```python
from build123d import *

# Parameters (mm, degrees)
SZKIC1_W = 9
SZKIC1_H = 21
SZKIC3_W = 1.2
SZKIC3_H = 2.1
SZKIC4_W = 6
SZKIC4_H = 23.5
SZKIC5_W = 40
SZKIC5_H = 21
SZKIC6_W = 1.2
SZKIC6_H = 2.1
SZKIC8_W = 165
SZKIC8_H = 16
SZKIC9_W = 1.2
SZKIC9_H = 1.6


with BuildPart() as part:
    # Szkic1 → Obr_t1 (revolve)
    with BuildSketch(Plane(origin=(0, 0, 0), x_dir=(0, 0, -1), z_dir=(1, 0, 0)), mode=Mode.PRIVATE) as obr_t1_sk:
        with Locations((-4.5, 10.5)):
            Rectangle(SZKIC1_W, SZKIC1_H)
    revolve(obr_t1_sk.sketch.rotate(Axis((0, 0, 0), (0, 0, 1)), 270), axis=Axis((0, 0, 0), (0, 0, 1)))

    # Szkic2 → Wyci_cie-obr_t1 (revolve, cut)
    with BuildSketch(Plane(origin=(0, 0, 0), x_dir=(0, 0, -1), z_dir=(1, 0, 0)), mode=Mode.PRIVATE) as wyci_cie_obr_t1_sk:
        Polygon((-0.707106781, 21), (0, 20.292893219), (0, 21), align=None)
    revolve(wyci_cie_obr_t1_sk.sketch.rotate(Axis((0, 0, 0), (0, 0, 1)), 270), axis=Axis((0, 0, 0), (0, 0, 1)), mode=Mode.SUBTRACT)

    # Szkic3 → Wyci_cie-obr_t2 (revolve, cut)
    with BuildSketch(Plane(origin=(0, 0, 0), x_dir=(0, 0, -1), z_dir=(1, 0, 0)), mode=Mode.PRIVATE) as wyci_cie_obr_t2_sk:
        with Locations((-8.4, 19.95)):
            Rectangle(SZKIC3_W, SZKIC3_H)
    revolve(wyci_cie_obr_t2_sk.sketch.rotate(Axis((0, 0, 0), (0, 0, 1)), 270), axis=Axis((0, 0, 0), (0, 0, 1)), mode=Mode.SUBTRACT)

    # Szkic4 → Obr_t2 (revolve)
    with BuildSketch(Plane(origin=(0, 0, 0), x_dir=(0, 0, -1), z_dir=(1, 0, 0)), mode=Mode.PRIVATE) as obr_t2_sk:
        with Locations((-12, 11.75)):
            Rectangle(SZKIC4_W, SZKIC4_H)
    revolve(obr_t2_sk.sketch.rotate(Axis((0, 0, 9), (0, 0, 1)), 270), axis=Axis((0, 0, 9), (0, 0, 1)))

    # Szkic5 → Obr_t3 (revolve)
    with BuildSketch(Plane(origin=(0, 0, 0), x_dir=(0, 0, -1), z_dir=(1, 0, 0)), mode=Mode.PRIVATE) as obr_t3_sk:
        with Locations((-35, 10.5)):
            Rectangle(SZKIC5_W, SZKIC5_H)
    revolve(obr_t3_sk.sketch.rotate(Axis((0, 0, 15), (0, 0, 1)), 270), axis=Axis((0, 0, 15), (0, 0, 1)))

    # Szkic6 → Wyci_cie-obr_t3 (revolve, cut)
    with BuildSketch(Plane(origin=(0, 0, 0), x_dir=(0, 0, -1), z_dir=(1, 0, 0)), mode=Mode.PRIVATE) as wyci_cie_obr_t3_sk:
        with Locations((-15.6, 19.95)):
            Rectangle(SZKIC6_W, SZKIC6_H)
    revolve(wyci_cie_obr_t3_sk.sketch.rotate(Axis((0, 0, 15), (0, 0, 1)), 270), axis=Axis((0, 0, 15), (0, 0, 1)), mode=Mode.SUBTRACT)

    # Szkic7 → Wyci_cie-obr_t4 (revolve, cut)
    with BuildSketch(Plane(origin=(0, 0, 0), x_dir=(0, 0, -1), z_dir=(1, 0, 0)), mode=Mode.PRIVATE) as wyci_cie_obr_t4_sk:
        Polygon((-55, 20.292893219), (-54.292893219, 21), (-55, 21), align=None)
    revolve(wyci_cie_obr_t4_sk.sketch.rotate(Axis((0, 0, 9), (0, 0, 1)), 270), axis=Axis((0, 0, 9), (0, 0, 1)), mode=Mode.SUBTRACT)

    # Szkic8 → Obr_t4 (revolve)
    with BuildSketch(Plane(origin=(0, 0, 0), x_dir=(0, 0, -1), z_dir=(1, 0, 0)), mode=Mode.PRIVATE) as obr_t4_sk:
        with Locations((-137.5, 8)):
            Rectangle(SZKIC8_W, SZKIC8_H)
    revolve(obr_t4_sk.sketch.rotate(Axis((0, 0, 55), (0, 0, 1)), 270), axis=Axis((0, 0, 55), (0, 0, 1)))

    # Szkic9 → Wyci_cie-obr_t5 (revolve, cut)
    with BuildSketch(Plane(origin=(0, 0, 0), x_dir=(0, 0, -1), z_dir=(1, 0, 0)), mode=Mode.PRIVATE) as wyci_cie_obr_t5_sk:
        with Locations((-55.6, 15.2)):
            Rectangle(SZKIC9_W, SZKIC9_H)
    revolve(wyci_cie_obr_t5_sk.sketch.rotate(Axis((0, 0, 55), (0, 0, 1)), 270), axis=Axis((0, 0, 55), (0, 0, 1)), mode=Mode.SUBTRACT)

    # Szkic10 → Wyci_cie-obr_t6 (revolve, cut)
    with BuildSketch(Plane(origin=(0, 0, 0), x_dir=(0, 0, -1), z_dir=(1, 0, 0)), mode=Mode.PRIVATE) as wyci_cie_obr_t6_sk:
        Polygon((-220, 14.124355653), (-213, 16), (-220, 16), align=None)
    revolve(wyci_cie_obr_t6_sk.sketch.rotate(Axis((0, 0, 55), (0, 0, 1)), 270), axis=Axis((0, 0, 55), (0, 0, 1)), mode=Mode.SUBTRACT)

    # Szkic11 → Wyci_cie-obr_t7 (revolve, cut)
    with BuildSketch(Plane(origin=(0, 0, 0), x_dir=(0, 0, -1), z_dir=(1, 0, 0)), mode=Mode.PRIVATE) as wyci_cie_obr_t7_sk:
        with BuildLine():
            Line((-218.332342851, 14.571203039), (-220, 14.124355653))
            Line((-220, 14.124355653), (-220, 12.39786993))
            ThreePointArc((-220, 12.39786993), (-219.535045016, 13.767583145), (-218.332342851, 14.571203039))
        make_face()
    revolve(wyci_cie_obr_t7_sk.sketch.rotate(Axis((0, 0, 55), (0, 0, 1)), 270), axis=Axis((0, 0, 55), (0, 0, 1)), mode=Mode.SUBTRACT)

    # Szkic12 → Wyci_cie-obr_t8 (revolve, cut)
    with BuildSketch(Plane(origin=(0, 0, 0), x_dir=(0, 0, -1), z_dir=(1, 0, 0)), mode=Mode.PRIVATE) as wyci_cie_obr_t8_sk:
        with BuildLine():
            Line((-172.257142857, 16), (-173.457142857, 16))
            ThreePointArc((-173.457142857, 16), (-172.857142857, 15.4), (-172.257142857, 16))
        make_face()
    revolve(wyci_cie_obr_t8_sk.sketch.rotate(Axis((0, 0, 172.257142857), (0, 0, 1)), 270), axis=Axis((0, 0, 172.257142857), (0, 0, 1)), mode=Mode.SUBTRACT)

    # Szkic13 → Wyci_cie-obr_t9 (revolve, cut)
    with BuildSketch(Plane(origin=(0, 0, 0), x_dir=(0, 0, -1), z_dir=(1, 0, 0)), mode=Mode.PRIVATE) as wyci_cie_obr_t9_sk:
        with BuildLine():
            Line((-113.328570957, 16), (-114.528570957, 16))
            ThreePointArc((-114.528570957, 16), (-113.928570957, 15.4), (-113.328570957, 16))
        make_face()
    revolve(wyci_cie_obr_t9_sk.sketch.rotate(Axis((0, 0, 113.328570957), (0, 0, 1)), 270), axis=Axis((0, 0, 113.328570957), (0, 0, 1)), mode=Mode.SUBTRACT)


solid = part.part
```
Can you work these out from the model? Positions are in its coordinate system, mm. A direction names the side the tool comes from. Give positions to 0.01 mm unless a question says otherwise; leave off trailing zeros. Loops run counter-clockwise (first coordinate to the right, second up) from the corner with the lowest first, then second, coordinate; pieces in that order, holes last. Notation, with made-up numbers: M 38,21 L 86,21 A33 cw 86,54 Z; hole C 8.5,41 d6. An arc over 180 degrees is marked long. Answer in a Markdown table with one row per item.
1. Thinking about a two-plate mould opening in Z: for faces 5 (the flat face through (0, 0, 220)), 6 (the cylindrical face through (-3.47, -15.62, 84.36)), 7 (the flat face through (19, 3, 16.2)), 8 (the flat face through (16, 11, 9)), which applies, released by +Z, released by -Z, zero draft, split by the parting line, or undercut?
Taken from the geometry:
| item | result |
|---|---|
| face 5 | released by +Z |
| face 6 | zero draft |
| face 7 | undercut |
| face 8 | undercut |
2. Suppose I cut it at A-A on z = 24.5. Write out the boundary of the cut face in (x, y), plus the area to 3 significant figures.
Taken from the geometry:
| item | result |
|---|---|
| outline | C 0,0 d42 |
| area | 1,390 mm² |
3. For pin 1 Ø12 at (x, z) = (11.5, 84.5) entering from -Y (3 decimals); pin 2 Ø1.5 at (y, z) = (5, 109.5) entering from +X; pin 3 Ø5 at (x, y) = (6, 8) entering from -Z; pin 4 Ø12 at (x, z) = (18, 30) entering from -Y, each with a flat end and sliding along its axis, tell me the tip position at first contact or that it passes through.
Taken from the geometry:
| item | result |
|---|---|
| pin 1 | stops at y = -15.025 |
| pin 2 | stops at x = 15.43 |
| pin 3 | stops at z = 0 |
| pin 4 | stops at y = -17.23 |
4. Which directions (+Z, -Z, +X, -X, +Y, -Y) give clear straight access to the entire face, cutting with the end or side of a thin tool? Please do faces 1 (the cylindrical face through (20.03, 6.31, 4.2)), 2 (the cylindrical face through (-3.47, -15.62, 142.99)), 3 (the flat face through (19, 3, 7.8)), 4 (the flat face through (0, 0, 0)).
Taken from the geometry:
| item | result |
|---|---|
| face 1 | -Z |
| face 2 | +Z |
| face 3 | none |
| face 4 | -Z, +X, -X, +Y, -Y |
5. Suppose I cut it at B-B on z = 137.5. Write out the boundary of the cut face in (x, y), plus the area to 3 significant figures.
Taken from the geometry:
| item | result |
|---|---|
| outline | C 0,0 d32 |
| area | 804 mm² |
6. If I drill on line 1 along Z through (x, y) = (8, -19); line 2 along Y through (x, z) = (7, 194); line 3 along Z through (x, y) = (-17, -8), over which ranges is the centre line in solid material (lowest first)?
Taken from the geometry:
| item | result |
|---|---|
| line 1 | z = 0.32 to 7.8, 9 to 15, 16.2 to 54.68 |
| line 2 | y = -14.39 to 14.39 |
| line 3 | z = 0 to 55 |
